Source: CAD feature listing. Evaluate the final solid. Frame: model axes, mm. Face numbers are marked on the shaded views. A direction names the side the tool comes from. Give positions to 0.01 mm unless a question says otherwise; leave off trailing zeros. Order: outer loops, then holes, each group sorted by start corner. A loop starts at its lowest first (then second) coordinate and runs counter-clockwise, first axis right, second up. Notation, with made-up numbers: (-36, -8) -> (-28, -8) arc R28 cw to (-28, 15) -> close; hole circle Ø3 at (86, -9.5). An arc over 180 degrees is marked (long way). Answer in a Markdown table with one row per item.
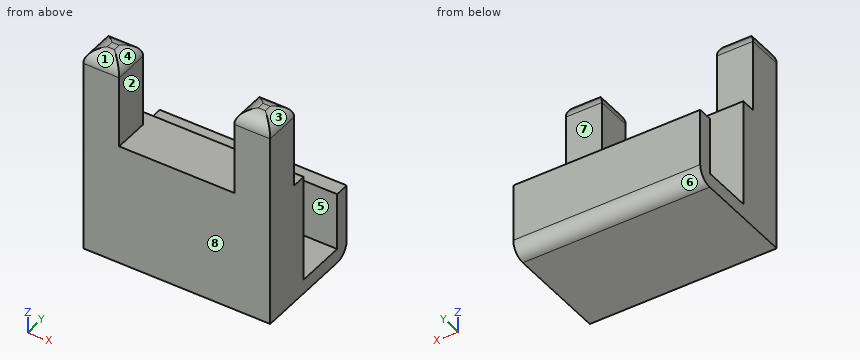
```python
from build123d import *

# Parameters (mm, degrees)
F0_W     = 26
F0_H     = 16
F1_DEPTH = 2
F2_W     = 26
F2_H     = 7
F3_DEPTH = 15
F2_H_2   = 2
F4_DEPTH = 8
F5_W     = 5
F5_H     = 5
F6_DEPTH = 12
F7_R     = 2
F8_R     = 2


with BuildPart() as f1:
    # F0 (on Top) → F1 (new body)
    with BuildSketch(Plane.XY):
        with Locations((-13, 8)):
            Rectangle(F0_W, F0_H)
    extrude(amount=F1_DEPTH)

    # F2 (on face) → F3 (join)
    with BuildSketch(Plane.XY.offset(2)):
        with Locations((-13, 3.5)):
            Rectangle(F2_W, F2_H)
    extrude(amount=F3_DEPTH)

    # F2 (on face) → F4 (join)
    with BuildSketch(Plane.XY.offset(2)):
        with Locations((-13, 15)):
            Rectangle(F2_W, F2_H_2)
    extrude(amount=F4_DEPTH)

    # F5 (on face) → F6 (join)
    with BuildSketch(Plane.XY.offset(17)):
        with Locations((-23.5, 2.5)):
            Rectangle(F5_W, F5_H)
        with Locations((-2.5, 2.5)):
            Rectangle(F5_W, F5_H)
    extrude(amount=F6_DEPTH)

    # F7
    f7_edges = [f1.edges().sort_by_distance(p)[0] for p in [
        (-13, 16, 0),
    ]]
    fillet(f7_edges, radius=F7_R)

    # F8
    f8_edges = [f1.edges().sort_by_distance(p)[0] for p in [
        (-26, 2.5, 29),
        (-23.5, 0, 29),
        (-21, 2.5, 29),
        (-23.5, 5, 29),
        (-2.5, 0, 29),
        (0, 2.5, 29),
        (-2.5, 5, 29),
        (-5, 2.5, 29),
    ]]
    fillet(f8_edges, radius=F8_R)


solid = f1.part
```
(1) Access query for the marked faces 4, 5, 6, 7 and 8. Directions: +Z, -Z, +X, -X, +Y, -Y. A direction counts if a zero-diameter tool reaches every point of the face in a straight line with its end or side. Return the directions, or none.
A:
| item | result |
|---|---|
| face 4 | +Z, +Y, -Y |
| face 5 | +Z, +X, -X |
| face 6 | -Z, +X, -X, +Y |
| face 7 | +Z, +X, -X, +Y |
| face 8 | +Z, -Z, +X, -X, -Y |
(2) Section query B-B (x = -12.75). Return the cut outline in (y, z), plus the area to 3 significant figures.
A:
| item | result |
|---|---|
| outline | (0, 0) -> (14, 0) arc R2 ccw to (16, 2) -> (16, 10) -> (14, 10) -> (14, 2) -> (7, 2) -> (7, 17) -> (0, 17) -> close |
| area | 152 mm^2 |
(3) Section query C-C (y = 3.5). Return the cut outline in (x, z).
A:
| item | result |
|---|---|
| outline | (-26, 0) -> (0, 0) -> (0, 27) arc R2 ccw to (-1.5, 28.94) -> (-3.5, 28.94) arc R2 ccw to (-5, 27) -> (-5, 17) -> (-21, 17) -> (-21, 27) arc R2 ccw to (-22.5, 28.94) -> (-24.5, 28.94) arc R2 ccw to (-26, 27) -> close |
(4) Section query A-A (z = 19.5). Return the cut outline in (x, y), plus the area to 3 significant figures.
A:
| item | result |
|---|---|
| outline | (-26, 0) -> (-21, 0) -> (-21, 5) -> (-26, 5) -> close; (-5, 0) -> (0, 0) -> (0, 5) -> (-5, 5) -> close |
| area | 50.0 mm^2 |
(5) Pull-direction query (X, two-part tool) for the marked faces 1, 2 and 3; classes: +X half, -X half, draft (parallel to the pull), parting line (faces both ways), or undercut.
A:
| item | result |
|---|---|
| face 1 | draft |
| face 2 | undercut |
| face 3 | +X half |
(6) Ray query, probe 1 along Y at (x, z) = (-20.5, 3); probe 2 along X at (y, z) = (3, 22.5); probe 3 along Z at (x, y) = (-18.5, 9.5). Return the intervals inside material, ascending.
A:
| item | result |
|---|---|
| probe 1 | y = 0 to 7, 14 to 16 |
| probe 2 | x = -26 to -21, -5 to 0 |
| probe 3 | z = 0 to 2 |
(7) First-contact query: pin 1 Ø7.5 at (x, y) = (-19.5, 10) entering from +Z; pin 2 Ø1.5 at (x, z) = (-23, 21.5) entering from +Y; pin 3 Ø2 at (x, y) = (-17.5, 15) entering from +Z. Flat tips, straight axial feed; report the tip coordinate or a pass-through.
A:
| item | result |
|---|---|
| pin 1 | stops at z = 17 |
| pin 2 | stops at y = 5 |
| pin 3 | stops at z = 10 |
(8) Section query D-D (z = 4.5). Return the cut outline in (x, y).
A:
| item | result |
|---|---|
| outline | (-26, 0) -> (0, 0) -> (0, 7) -> (-26, 7) -> close; (-26, 14) -> (0, 14) -> (0, 16) -> (-26, 16) -> close |
